Verification items for the finished model (mm, model axes). A direction names the side the tool comes from. Give positions to 0.01 mm unless a question says otherwise; leave off trailing zeros. Loops run counter-clockwise (first coordinate to the right, second up) from the corner with the lowest first, then second, coordinate; pieces in that order, holes last. Notation, with made-up numbers: (-0.75, 79) - (17.25, 79) arc R24 ccw to (17.25, 96) - close; hole circle Ø10 at (51.25, -9). An arc over 180 degrees is marked (long way). Answer in a Markdown table with one row per item.
```python
from build123d import *

# Parameters (mm, degrees)
SKETCH005_R  = 1.5
PAD004_DEPTH = 22
SKETCH004_W  = 8
SKETCH004_H  = 38
PAD003_DEPTH = 22
SKETCH006_R  = 2.3
PAD005_DEPTH = 70
SKETCH002_W  = 160
SKETCH002_H  = 40
PAD002_DEPTH = 40
SKETCH_R     = 10
PAD001_DEPTH = 5
SKETCH001_W  = 160
SKETCH001_H  = 40
PAD_DEPTH    = 3
PAD006_DEPTH = 20


with BuildPart() as pylon_thread_holes:
    # Sketch005 → Pad004 (new body)
    with BuildSketch(Plane.XY):
        with Locations((-68.335, 10.855)):
            Circle(SKETCH005_R)
        with Locations((-31.665, 10.855)):
            Circle(SKETCH005_R)
        with Locations((-68.335, -10.855)):
            Circle(SKETCH005_R)
        with Locations((-31.665, -10.855)):
            Circle(SKETCH005_R)
        with Locations((31.665, 10.855)):
            Circle(SKETCH005_R)
        with Locations((31.665, -10.855)):
            Circle(SKETCH005_R)
        with Locations((68.335, 10.855)):
            Circle(SKETCH005_R)
        with Locations((68.335, -10.855)):
            Circle(SKETCH005_R)
    extrude(amount=PAD004_DEPTH)


with BuildPart() as pylons:
    # Sketch004 → Pad003 (new body)
    with BuildSketch(Plane.XY):
        with Locations((-68.335, 0)):
            Rectangle(SKETCH004_W, SKETCH004_H)
        with Locations((-31.665, 0)):
            Rectangle(SKETCH004_W, SKETCH004_H)
        with Locations((31.665, 0)):
            Rectangle(SKETCH004_W, SKETCH004_H)
        with Locations((68.335, 0)):
            Rectangle(SKETCH004_W, SKETCH004_H)
    extrude(amount=PAD003_DEPTH)

    # Cut001: cut Pylon Thread Holes
    add(pylon_thread_holes.part, mode=Mode.SUBTRACT)


with BuildPart() as back_panel_screw_holes:
    # Sketch006 → Pad005 (new body)
    with BuildSketch(Plane.XY):
        with Locations((-76, 16)):
            Circle(SKETCH006_R)
        with Locations((-76, -16)):
            Circle(SKETCH006_R)
        with Locations((76, 16)):
            Circle(SKETCH006_R)
        with Locations((76, -16)):
            Circle(SKETCH006_R)
    extrude(amount=PAD005_DEPTH)


with BuildPart() as sidewall:
    # Sketch002 → Pad002 (new body)
    with BuildSketch(Plane.XY):
        Rectangle(SKETCH002_W, SKETCH002_H)
        with BuildLine():
            Line((75, 8.254033), (75, -8))
            ThreePointArc((67, -16), (72.656854, -13.656854), (75, -8))
            Line((67, -16), (-67, -16))
            ThreePointArc((-75, -8), (-72.656854, -13.656854), (-67, -16))
            Line((-75, -8), (-75, 8.254033))
            ThreePointArc((-69, 16), (-73.324555, 13.153013), (-75, 8.254033))
            Line((-69, 16), (69, 16))
            ThreePointArc((75, 8.254033), (73.324555, 13.153013), (69, 16))
        make_face(mode=Mode.SUBTRACT)
    extrude(amount=PAD002_DEPTH)

    # Cut002: cut Back Panel Screw Holes
    add(back_panel_screw_holes.part, mode=Mode.SUBTRACT)


with BuildPart() as lens_holes:
    # Sketch → Pad001 (new body)
    with BuildSketch(Plane.XY):
        with Locations((-50, 0)):
            Circle(SKETCH_R)
        with Locations((50, 0)):
            Circle(SKETCH_R)
    extrude(amount=PAD001_DEPTH)


with BuildPart() as whole:
    # Sketch001 → Pad (new body)
    with BuildSketch(Plane.XY):
        Rectangle(SKETCH001_W, SKETCH001_H)
    extrude(amount=PAD_DEPTH)

    # Cut: cut Lens Holes
    add(lens_holes.part, mode=Mode.SUBTRACT)

    # Fusion: union Sidewall
    add(sidewall.part)

    # Fusion001: union Pylons
    add(pylons.part)


with BuildPart() as fusion002:
    # Sketch007 → Pad006 (new body)
    with BuildSketch(Plane.XY):
        Polygon((-21.12132, 19), (-2.12132, 0), (-21.12132, -19), (-16.87868, -19), (0, -2.12132), (16.87868, -19), (21.12132, -19), (2.12132, 0), (21.12132, 19), (16.87868, 19), (0, 2.12132), (-16.87868, 19), align=None)
    extrude(amount=PAD006_DEPTH)

    # Fusion002: union Whole
    add(whole.part)


solid = fusion002.part
```
Q1. Thickness scan on line 1 (Y direction, x = -25, z = 10.5); line 2 (Y direction, x = 76, z = 15); line 3 (X direction, y = 0, z = 1.25). Record the ranges inside material, lowest first.
Completed:
| item | result |
|---|---|
| line 1 | -20 to -16, 16 to 20 |
| line 2 | -20 to -18.3, -13.7 to 13.7, 18.3 to 20 |
| line 3 | -80 to -60, -40 to 40, 60 to 80 |
Q2. Sectioned sample at C-C (x = -61.5). Record the cut outline in (y, z).
Completed:
| item | result |
|---|---|
| outline | (-20, 0) - (20, 0) - (20, 40) - (16, 40) - (16, 3) - (-16, 3) - (-16, 40) - (-20, 40) - close |
Q3. Sectioned sample at A-A (z = 29). Record the cut outline in (x, y).
Completed:
| item | result |
|---|---|
| outline | (-80, -20) - (80, -20) - (80, 20) - (-80, 20) - close; hole circle Ø4.6 at (-76, -16); hole circle Ø4.6 at (-76, 16); hole (-75, -8) arc R8 ccw to (-67, -16) - (67, -16) arc R8 ccw to (75, -8) - (75, 8.25) arc R8 ccw to (69, 16) - (-69, 16) arc R8 ccw to (-75, 8.25) - close; hole circle Ø4.6 at (76, -16); hole circle Ø4.6 at (76, 16) |
Q4. Sectioned sample at D-D (y = 6). Give the number of separate pieces and of enclosed holes in the cut face, and give its area (3 significant figures).
Completed:
| item | result |
|---|---|
| separate pieces | 3 |
| enclosed holes | 0 |
| area | 1,510 mm^2 |
Q5. Draft check along Y on faces 1 (the face through (-27.665, 0, 12)), 2 (the face through (-1, -20, 20)), 3 (the face through (80, 0, 20)). Enter one of: +Y half, -Y half, draft (parallel to the pull), parting line (faces both ways), or undercut.
Completed:
| item | result |
|---|---|
| face 1 | undercut |
| face 2 | -Y half |
| face 3 | draft |
Q6. Sectioned sample at B-B (x = 50). Record the cut outline in (y, z).
Completed:
| item | result |
|---|---|
| outline | (-20, 0) - (-10, 0) - (-10, 3) - (-16, 3) - (-16, 40) - (-20, 40) - close; (10, 0) - (20, 0) - (20, 40) - (16, 40) - (16, 3) - (10, 3) - close |
Q7. Go/stop test with flat-tipped pins: P1, Ø4, axis at x = -2.5, y = 9, coming from the +Z side; P2, Ø15.5, axis at x = 3.5, y = -6.5, coming from the +Z side; P3, Ø2.5, axis at x = 67.5, y = -2.5, coming from the +Z side. Record where each tip stops, or that it passes through.
Completed:
| item | result |
|---|---|
| P1 | z = 3 |
| P2 | z = 20 |
| P3 | z = 22 |
Q8. Tool access check on faces 4 (the face through (-73.875, 15.119, 21.241)), 5 (the face through (-60, 0, 1)). Record the directions out of +Z, -Z, +X, -X, +Y, -Y that give a thin tool (end or side, any length) a straight path to the whole face; none if there is none.
Completed:
| item | result |
|---|---|
| face 4 | +Z |
| face 5 | +Z, -Z |
